from build123d import *

# Parameters (mm, degrees)
SKETCH1_W           = 450
SKETCH1_H           = 450
BOSS_EXTRUDE1_DEPTH = 50
SKETCH2_W           = 40
SKETCH2_H           = 40
BOSS_EXTRUDE2_DEPTH = 360
BOSS_EXTRUDE3_DEPTH = 600
SKETCH4_W           = 30
SKETCH4_H           = 520
CUT_EXTRUDE2_DEPTH  = 300
FILLET2_R           = 10
FILLET4_R           = 10


with BuildPart() as part:
    # Sketch1 → Boss-Extrude1 (new body)
    with BuildSketch(Plane(origin=(0, 0, 0), x_dir=(1, 0, 0), z_dir=(0, 1, 0))):
        Rectangle(SKETCH1_W, SKETCH1_H)
    extrude(amount=BOSS_EXTRUDE1_DEPTH)

    # Sketch2 → Boss-Extrude2 (add)
    with BuildSketch(Plane(origin=(0, 0, 0), x_dir=(-1, 0, 0), z_dir=(0, -1, 0))):
        Polygon((225, -225), (185.000000233, -225.004313347), (185.000000057, -185.004313347), (225, -185.002182787), align=None)
        Polygon((185.000923636, 225), (185, 185.000000011), (225, 185.000000011), (225, 225), align=None)
        with Locations((-205, 205)):
            Rectangle(SKETCH2_W, SKETCH2_H)
        with Locations((-205, -205)):
            Rectangle(SKETCH2_W, SKETCH2_H)
    extrude(amount=BOSS_EXTRUDE2_DEPTH)

    # Sketch3 → Boss-Extrude3 (add)
    with BuildSketch(Plane(origin=(0, 50, 0), x_dir=(1, 0, 0), z_dir=(0, 1, 0))):
        Polygon((-225, 225), (-225, 183.319526978), (225, 185.000000043), (225, 225), align=None)
    extrude(amount=BOSS_EXTRUDE3_DEPTH)

    # Sketch4 → Cut-Extrude2 (cut, symmetric)
    with BuildSketch(Plane(origin=(-0.687713792, 0, -184.157195323), x_dir=(0.999993027, 0, -0.003734359), z_dir=(0.003734359, 0, 0.999993027))):
        with Locations((-150.5, 310)):
            Rectangle(SKETCH4_W, SKETCH4_H)
        with Locations((89.5, 310)):
            Rectangle(SKETCH4_W, SKETCH4_H)
        with Locations((-90.5, 310)):
            Rectangle(SKETCH4_W, SKETCH4_H)
        with Locations((-30.5, 310)):
            Rectangle(SKETCH4_W, SKETCH4_H)
        with Locations((149.5, 310)):
            Rectangle(SKETCH4_W, SKETCH4_H)
        with Locations((29.5, 310)):
            Rectangle(SKETCH4_W, SKETCH4_H)
        Polygon((-164.5, 631.432523358), (164.5, 631.432523358), (164.5, 652.515401433), (-164.5, 650), align=None)
    extrude(amount=CUT_EXTRUDE2_DEPTH, both=True, mode=Mode.SUBTRACT)

    # Fillet2
    fillet2_edges = [part.edges().sort_by_distance(p)[0] for p in [
        (194.330455246, 650, -225),
        (225, 650, -205.000000022),
        (194.405569596, 650, -184.885748674),
        (163.736024842, 650, -204.885748652),
    ]]
    fillet(fillet2_edges, radius=FILLET2_R)

    # Fillet4
    fillet4_edges = [part.edges().sort_by_distance(p)[0] for p in [
        (-225, 650, -204.159763489),
        (-195.093283388, 650, -183.43121016),
        (-195.170691778, 650, -225),
        (-165.263975166, 650, -204.271446671),
    ]]
    fillet(fillet4_edges, radius=FILLET4_R)


solid = part.part
Source: CAD feature listing. Evaluate the final solid. Frame: model axes, mm. A direction names the side the tool comes from. Round coordinates to 2 decimals unless told otherwise and drop trailing zeros. Write each loop counter-clockwise with the first axis right and the second up, starting at its lowest first coordinate (ties: lowest second). Pieces come first, ordered by that corner, then holes. Notation, with made-up numbers: (12, 76) - (43, 76) arc R21 ccw to (43, 90) - close; hole circle Ø8 at (13.25, -3). An arc over 180 degrees is marked (long way). Use CSV: the item, a comma, the result in double quotes. Start each with the question number.
(1) Cut plane D-D, the plane x = 122.5. Return loops of the section in (y, z).
(2) Mould query, pull axis X, two halves, no side actions, for faces 1 (the face through (-205, -177, -185)), 2 (the face through (89, 570, -205)), 3 (the face through (-225, 27, -84)). Classes: pulls with the +X half, pulls with the -X half, needs draft (parallel to the pull), parting line crosses it, or undercut.
(3) First-contact query: pin 1 Ø12 at (x, z) = (138.5, -75.5) entering from +Y; pin 2 Ø24 at (x, z) = (142, -207) entering from -Y; pin 3 Ø1 at (x, y) = (-51, 529.5) entering from +Z. Flat tips, straight axial feed; report the tip coordinate or a pass-through.
(4) Set-up query: faces 4 (the face through (205, -360, -205)), 5 (the face through (185, -177, -205)). Return all of +Z, -Z, +X, -X, +Y, -Y with unobstructed straight access to the full face (end or side cutting, diameter ignored); none if empty.
(5) Cut plane A-A, the plane y = -222.5. Return loops of the section in (x, z).
(6) Cut plane B-B, the plane y = 539.5. Return loops of the section in (x, z), and give its area (3 significant figures).
(7) Cut plane C-C, the plane x = -36. Return loops of the section in (y, z).
(8) Material intervals for probe 1 along Y at (x, z) = (-141, -201); probe 2 along X at (y, z) = (-264, 194.5); probe 3 along Y at (x, z) = (203, -115.5), sorted ascending. Write a range as [from, to].
Geometry says:
1,outline,"(0, -225) - (631.43, -225) - (631.43, -184.62) - (50, -184.62) - (50, 225) - (0, 225) - close"
2,face 1,"needs draft"
2,face 2,"undercut"
2,face 3,"pulls with the -X half"
3,pin 1,"y = 50"
3,pin 2,"y = 0"
3,pin 3,"z = -183.97"
4,face 4,"+Z, -Z, +X, -X, -Y"
4,face 5,"+Z, -Z, -Y"
5,outline,"(-225, -225) - (-185, -225) - (-185, -185) - (-225, -185) - close; (-225, 185) - (-185, 185) - (-185, 225) - (-225, 225) - close; (185, -225) - (225, -225) - (225, -185) - (185, -185) - close; (185, 185) - (225, 185) - (225, 225) - (185, 225) - close"
6,outline,"(-225, -225) - (-166.34, -225) - (-166.19, -183.54) - (-225, -183.32) - close; (-136.34, -225) - (-106.34, -225) - (-106.19, -183.76) - (-136.19, -183.65) - close; (-76.34, -225) - (-46.34, -225) - (-46.19, -183.99) - (-76.19, -183.88) - close; (-16.34, -225) - (13.66, -225) - (13.81, -184.21) - (-16.19, -184.1) - close; (43.66, -225) - (73.66, -225) - (73.81, -184.44) - (43.81, -184.32) - close; (103.66, -225) - (133.66, -225) - (133.81, -184.66) - (103.81, -184.55) - close; (163.66, -225) - (225, -225) - (225, -185) - (163.81, -184.77) - close"
6,area,"11,000 mm²"
7,outline,"(0, -225) - (50, -225) - (50, 225) - (0, 225) - close; (570, -225) - (631.43, -225) - (631.43, -184.03) - (570, -184.03) - close"
8,probe 1,"[0, 50], [570, 631.43]"
8,probe 2,"[-225, -185], [185, 225]"
8,probe 3,"[0, 50]"
